from build123d import *

# Parameters (mm, degrees)
SKIZZE1_W                       = 50
SKIZZE1_H                       = 18
AUFSATZ_LINEAR_AUSTRAGEN1_DEPTH = 3
SKIZZE2_R                       = 1.55
SCHNITT_LINEAR_AUSTRAGEN1_DEPTH = 37.043046724
FASE1_SIZE                      = 0.4


with BuildPart() as part:
    # Skizze1 → Aufsatz-Linear austragen1 (new body)
    with BuildSketch(Plane.XY):
        with Locations((9.62254438, -0.559322034)):
            Rectangle(SKIZZE1_W, SKIZZE1_H)
    extrude(amount=AUFSATZ_LINEAR_AUSTRAGEN1_DEPTH)

    # Skizze2 → Schnitt-Linear austragen1 (cut, through all)
    with BuildSketch(Plane(origin=(0, 0, 0), x_dir=(-1, 0, 0), z_dir=(0, 0, -1))):
        with Locations((9.37745562, 4.440677966)):
            Circle(SKIZZE2_R)
        with Locations((-5.62254438, 4.440677966)):
            Circle(SKIZZE2_R)
        with Locations((-5.62254438, -5.559322034)):
            Circle(SKIZZE2_R)
        with Locations((9.37745562, -5.559322034)):
            Circle(SKIZZE2_R)
    extrude(amount=-SCHNITT_LINEAR_AUSTRAGEN1_DEPTH, mode=Mode.SUBTRACT)

    # Fase1
    fase1_edges = [part.edges().sort_by_distance(p)[0] for p in [
        (34.62254438, -0.559322034, 3),
        (9.62254438, 8.440677966, 3),
        (-7.82745562, -5.559322034, 3),
        (-7.82745562, -5.559322034, 0),
        (7.17254438, -5.559322034, 3),
        (7.17254438, -5.559322034, 0),
        (7.17254438, 4.440677966, 3),
        (7.17254438, 4.440677966, 0),
        (-7.82745562, 4.440677966, 3),
        (-7.82745562, 4.440677966, 0),
        (-15.37745562, -0.559322034, 3),
        (9.62254438, 8.440677966, 0),
        (34.62254438, -0.559322034, 0),
        (9.62254438, -9.559322034, 0),
        (-15.37745562, -0.559322034, 0),
        (-15.37745562, 8.440677966, 1.5),
        (34.62254438, 8.440677966, 1.5),
        (34.62254438, -9.559322034, 1.5),
        (-15.37745562, -9.559322034, 1.5),
        (9.62254438, -9.559322034, 3),
    ]]
    chamfer(fase1_edges, length=FASE1_SIZE)


solid = part.part
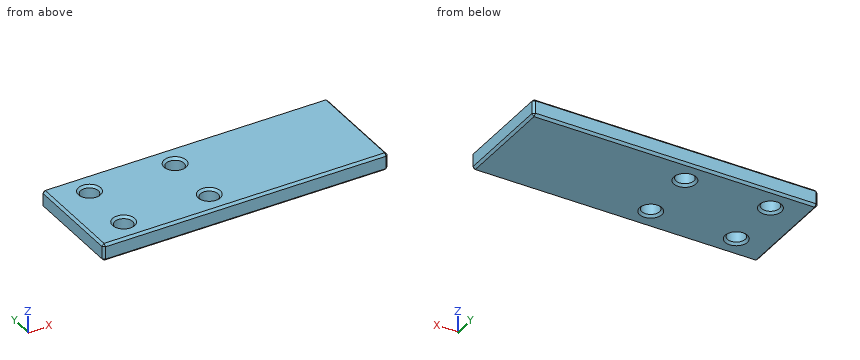
Can you work these out from the model? Positions are in its coordinate system, mm. Coordinates: 2 decimals unless noted, no trailing zeros. Loops run counter-clockwise (first coordinate to the right, second up) from the corner with the lowest first, then second, coordinate; pieces in that order, holes last. Notation, with made-up numbers: (31, -31.75) - (63, -31.75) arc R35 ccw to (63, 7.25) - close; hole circle Ø7 at (88, 16.5). An arc over 180 degrees is marked (long way). Put each result on its own line as item: value. Start each with the question number.
Item 1: Suppose I cut it at A-A (z = 0.9). Please give me the cut outline in (x, y).
Item 2: If I drill on line 1 along X through (y, z) = (-5.5, 2.5); line 2 along X through (y, z) = (-5, 0.9); line 3 along Y through (x, z) = (-8, 2.9), over which ranges is the centre line in solid material (lowest first)?
Item 3: Suppose I cut it at B-B (y = -6.25). State how many separate pieces and enclosed holes the cut face has, and give its area (3 significant figures).
Item 4: For pin 1 (3 mm diameter, centred on x = -9.38, y = -5.56, fed in from -Z); pin 2 (3.5 mm diameter, centred on x = 5.62, y = -5.56, fed in from +Z), each with a flat end and sliding along its axis, tell me the tip position at first contact or that it passes through.
Here are the results:
1. outline: (-15.38, -9.16) - (-14.98, -9.56) - (34.22, -9.56) - (34.62, -9.16) - (34.62, 8.04) - (34.22, 8.44) - (-14.98, 8.44) - (-15.38, 8.04) - close; hole circle Ø3.1 at (-9.38, -5.56); hole circle Ø3.1 at (-9.38, 4.44); hole circle Ø3.1 at (5.62, -5.56); hole circle Ø3.1 at (5.62, 4.44)
2. line 1: -15.38 to -10.93, -7.83 to 4.07, 7.17 to 34.62
2. line 2: -15.38 to -10.82, -7.93 to 4.18, 7.07 to 34.62
2. line 3: -9.26 to -6.79, -4.32 to 3.21, 5.68 to 8.14
3. separate pieces: 3
3. enclosed holes: 0
3. area: 132 mm²
4. pin 1: through
4. pin 2: z = 2.8
